```python
from build123d import *

# Parameters (mm, degrees)
F0_R      = 21.5
F1_DEPTH  = 35
F2_R      = 20
F3_DEPTH  = 25
F4_R      = 5
F5_DEPTH  = 2
F6_R      = 20
F7_DEPTH  = 6.5
F8_R      = 2
F9_R      = 5
F10_DEPTH = 2
F11_R     = 1
F12_R     = 2.5
F13_DEPTH = 16
F14_R     = 0.5
F15_R     = 1
F16_R     = 2.5
F17_DEPTH = 9.5


with BuildPart() as f1:
    # F0 (on Top) → F1 (new body)
    with BuildSketch(Plane.XY):
        Circle(F0_R)
    extrude(amount=-F1_DEPTH)

    # F2 (on face) → F3 (join)
    with BuildSketch(Plane.XY):
        Circle(F2_R)
    extrude(amount=F3_DEPTH)

    # F4 (on face) → F5 (join)
    with BuildSketch(Plane.XY.offset(25)):
        Circle(F4_R)
    extrude(amount=F5_DEPTH)

    # F6 (on face) → F7 (join)
    with BuildSketch(Plane(origin=(0, 0, -35), x_dir=(1, 0, 0), z_dir=(0, 0, -1))):
        Circle(F6_R)
    extrude(amount=F7_DEPTH)

    # F8
    f8_edges = [f1.edges().sort_by_distance(p)[0] for p in [
        (-20, 0, -41.5),
    ]]
    fillet(f8_edges, radius=F8_R)

    # F9 (on face) → F10 (join)
    with BuildSketch(Plane(origin=(0, 0, -41.5), x_dir=(1, 0, 0), z_dir=(0, 0, -1))):
        Circle(F9_R)
    extrude(amount=F10_DEPTH)

    # F11
    f11_edges = [f1.edges().sort_by_distance(p)[0] for p in [
        (-5, 0, -43.5),
    ]]
    fillet(f11_edges, radius=F11_R)

    # F12 (on face) → F13 (join)
    with BuildSketch(Plane(origin=(0, 0, -43.5), x_dir=(1, 0, 0), z_dir=(0, 0, -1))):
        Circle(F12_R)
    extrude(amount=F13_DEPTH)

    # F14
    f14_edges = [f1.edges().sort_by_distance(p)[0] for p in [
        (-2.5, 0, -59.5),
    ]]
    fillet(f14_edges, radius=F14_R)

    # F15
    f15_edges = [f1.edges().sort_by_distance(p)[0] for p in [
        (-5, 0, 27),
    ]]
    fillet(f15_edges, radius=F15_R)

    # F16 (on face) → F17 (join)
    with BuildSketch(Plane.XY.offset(27)):
        Circle(F16_R)
    extrude(amount=F17_DEPTH)


solid = f1.part
```
CAD build for the part. Positions are in the model's coordinates, mm. A direction names the side the tool comes from. Coordinates: 2 decimals unless noted, no trailing zeros. Order: outer loops, then holes, each group sorted by start corner. A loop starts at its lowest first (then second) coordinate and runs counter-clockwise, first axis right, second up.
(1) Saw through at A-A, the plane z = -46. Write the cut outline in (x, y), and give its area (3 significant figures).
Solution:
outline: circle Ø5 at (0, 0)
area: 19.6 mm2
(2) Pin check, flat tips, straight feed: pin 1 Ø5 at (y, z) = (-4.5, -26) entering from -X; pin 2 Ø4 at (x, z) = (-3, -10.5) entering from -Y; pin 3 Ø10 at (x, y) = (-3.5, -15.5) entering from +Z. Stop position of each tip, or through.
Solution:
pin 1: stops at x = -21.41
pin 2: stops at y = -21.48
pin 3: stops at z = 25
(3) Which spindle directions (+Z, -Z, +X, -X, +Y, -Y) get a long thin tool onto all of the face, cutting with end or side? Do faces 1 (the face through (0, 0, -59.5)), 2 (the face through (-4.336, 19.524, -37.218)), 3 (the face through (2, 2, 27)). Say none if no direction does.
Solution:
face 1: -Z, +X, -X, +Y, -Y
face 2: -Z
face 3: +Z
(4) Drill centre lines: L1, parallel to Z at x = 11, y = 1; L2, parallel to Z at x = -10.5, y = 18.5; L3, parallel to Y at x = 0, z = 14.5. Where is each one in solid material? Low to high.
Solution:
L1: z = -41.5 to 25
L2: z = -35 to 0
L3: y = -20 to 20
(5) Saw through at B-B, the plane z = -34. Write the cut outline in (x, y).
Solution:
outline: circle Ø43 at (0, 0)
